from build123d import *

# Parameters (mm, degrees)
SKETCH_1_W          = 30
SKETCH_1_H          = 750
SKETCH_1_R          = 2
EXTRUDE_2_DEPTH     = 70
SKETCH_2_W          = 26
SKETCH_2_H          = 66
CUT_EXTRUDE_3_DEPTH = 754.408919512
CUT_EXTRUDE_4_DEPTH = 382.772183376
SKETCH_8_R          = 3
SKETCH_8_R_2        = 2
CUT_EXTRUDE_6_DEPTH = 382.772183376
SKETCH_9_R          = 5.5
CUT_EXTRUDE_7_DEPTH = 316


with BuildPart() as part:
    # 草图1 → 凸台-拉伸2 (new body)
    with BuildSketch(Plane.XY):
        Rectangle(SKETCH_1_W, SKETCH_1_H)
        with Locations((-7.5, 194.978117754)):
            Circle(SKETCH_1_R, mode=Mode.SUBTRACT)
        with Locations((7.5, 194.978117754)):
            Circle(SKETCH_1_R, mode=Mode.SUBTRACT)
        with Locations((-7.5, 178.773554479)):
            Circle(SKETCH_1_R, mode=Mode.SUBTRACT)
        with Locations((7.5, 178.773554479)):
            Circle(SKETCH_1_R, mode=Mode.SUBTRACT)
        with Locations((-7.5, -150.877478615)):
            Circle(SKETCH_1_R, mode=Mode.SUBTRACT)
        with Locations((7.5, -150.877478615)):
            Circle(SKETCH_1_R, mode=Mode.SUBTRACT)
        with Locations((-7.5, -167.08204189)):
            Circle(SKETCH_1_R, mode=Mode.SUBTRACT)
        with Locations((7.5, -167.08204189)):
            Circle(SKETCH_1_R, mode=Mode.SUBTRACT)
    extrude(amount=EXTRUDE_2_DEPTH)

    # 草图2 → 切除-拉伸3 (cut, through all)
    with BuildSketch(Plane.XZ.offset(375)):
        with Locations((0, 35)):
            Rectangle(SKETCH_2_W, SKETCH_2_H)
    extrude(amount=-CUT_EXTRUDE_3_DEPTH, mode=Mode.SUBTRACT)

    # 草图3 → 切除-拉伸4 (cut, through all)
    with BuildSketch(Plane.XY.offset(70)):
        Polygon((15, -375), (15, -347.1), (-15, -343.150425072), (-15, -375), align=None)
        Polygon((15, 377.040830045), (15, 375), (-15, 371.050425072), (-15, 377.040830045), align=None)
    extrude(amount=-CUT_EXTRUDE_4_DEPTH, mode=Mode.SUBTRACT)

    # 草图8 → 切除-拉伸6 (cut, through all)
    with BuildSketch(Plane(origin=(0, 0, 0), x_dir=(-1, 0, 0), z_dir=(0, 0, -1))):
        with Locations((6.5, 364.870363851)):
            Circle(SKETCH_8_R)
        with Locations((-6.5, 364.870363851)):
            Circle(SKETCH_8_R)
        with Locations((-6.5, 344.870363851)):
            Circle(SKETCH_8_R)
        with Locations((6.5, 344.870363851)):
            Circle(SKETCH_8_R)
        with Locations((-7.5, -150.877478615)):
            Circle(SKETCH_8_R)
        with Locations((-7.5, -150.877478615)):
            Circle(SKETCH_8_R_2, mode=Mode.SUBTRACT)
        with Locations((7.5, -150.877478615)):
            Circle(SKETCH_8_R)
        with Locations((7.5, -150.877478615)):
            Circle(SKETCH_8_R_2, mode=Mode.SUBTRACT)
        with Locations((7.5, -167.08204189)):
            Circle(SKETCH_8_R)
        with Locations((7.5, -167.08204189)):
            Circle(SKETCH_8_R_2, mode=Mode.SUBTRACT)
        with Locations((-7.5, -167.08204189)):
            Circle(SKETCH_8_R)
        with Locations((-7.5, -167.08204189)):
            Circle(SKETCH_8_R_2, mode=Mode.SUBTRACT)
        with Locations((-7.49999999, 21.448037931)):
            Circle(SKETCH_8_R)
        with Locations((7.50000001, 21.448037931)):
            Circle(SKETCH_8_R)
        with Locations((-7.49999999, 6.448037931)):
            Circle(SKETCH_8_R)
        with Locations((7.50000001, 6.448037931)):
            Circle(SKETCH_8_R)
        with Locations((-7.5, 194.978117754)):
            Circle(SKETCH_8_R)
        with Locations((-7.5, 194.978117754)):
            Circle(SKETCH_8_R_2, mode=Mode.SUBTRACT)
        with Locations((-7.5, 178.773554479)):
            Circle(SKETCH_8_R)
        with Locations((-7.5, 178.773554479)):
            Circle(SKETCH_8_R_2, mode=Mode.SUBTRACT)
        with Locations((7.5, 194.978117754)):
            Circle(SKETCH_8_R)
        with Locations((7.5, 194.978117754)):
            Circle(SKETCH_8_R_2, mode=Mode.SUBTRACT)
        with Locations((7.5, 178.773554479)):
            Circle(SKETCH_8_R)
        with Locations((7.5, 178.773554479)):
            Circle(SKETCH_8_R_2, mode=Mode.SUBTRACT)
        with Locations((6.5, -316.970363851)):
            Circle(SKETCH_8_R)
        with Locations((-6.5, -316.970363851)):
            Circle(SKETCH_8_R)
        with Locations((-6.5, -336.970363851)):
            Circle(SKETCH_8_R)
        with Locations((6.5, -336.970363851)):
            Circle(SKETCH_8_R)
    extrude(amount=-CUT_EXTRUDE_6_DEPTH, mode=Mode.SUBTRACT)

    # 草图9 → 切除-拉伸7 (cut)
    with BuildSketch(Plane.XY.offset(70)):
        with Locations((-0.612697266, 155.502325872)):
            Circle(SKETCH_9_R)
        with Locations((-0.612697266, 221.502325872)):
            Circle(SKETCH_9_R)
    extrude(amount=-CUT_EXTRUDE_7_DEPTH, mode=Mode.SUBTRACT)


solid = part.part
Work out the finished part from the listing and answer in its coordinate system (mm). A direction names the side the tool comes from. Coordinates: 2 decimals unless noted, no trailing zeros. Write each loop counter-clockwise with the first axis right and the second up, starting at its lowest first coordinate (ties: lowest second). Pieces come first, ordered by that corner, then holes.
1. Consider line 1 along X through (y, z) = (219.5, 31); line 2 along Z through (x, y) = (5, 321.5); line 3 along Y through (x, z) = (13.5, 62). Determine where each line is inside the solid, lowest interval first.
Results list:
line 1: x = -15 to -13, 13 to 15
line 2: z = 0 to 2, 68 to 70
line 3: y = -346.9 to 374.8
2. For faces 5 (the flat face through (13.4, 374.79, 37.76)), 6 (the flat face through (0, 9, 68)), determine the directions among +Z, -Z, +X, -X, +Y, -Y from which every point of the face is accessible in a straight line to the end or side of a thin tool.
Results list:
face 5: +Z, -Z, -X, +Y
face 6: +Y, -Y
3. The part is cut by section B-B, the plane y = -253.5. Write down the section's boundary in (x, z), and give its area (3 significant figures).
Results list:
outline: (-15, 0) - (15, 0) - (15, 70) - (-15, 70) - close; hole (-13, 2) - (13, 2) - (13, 68) - (-13, 68) - close
area: 384 mm2
4. The part is cut by section A-A, the plane z = 36.5. Write down the section's boundary in (x, y), and give its area (3 significant figures).
Results list:
outline: (-15, -343.15) - (-13, -343.41) - (-13, 371.31) - (-15, 371.05) - close; (13, -346.84) - (15, -347.1) - (15, 375) - (13, 374.74) - close
area: 2,870 mm2
5. For a pull along Z with two mould halves and no side action, classify faces 1 (the flat face through (0, 19, 70)), 2 (the flat face through (0, 9, 2)), 3 (the flat face through (-13, 9, 35)), 4 (the cylindrical face through (-4.666, 159.219, 69.014)) as +Z half, -Z half, draft (parallel to the pull), parting line (faces both ways), or undercut.
Results list:
face 1: +Z half
face 2: undercut
face 3: undercut
face 4: draft
